Autodesk Inventor part; units mm, degrees
ref_plane "YZ Plane" through (0, 0, 0) normal (1, 0, 0) x (0, 1, 0)
ref_plane "XZ Plane" through (0, 0, 0) normal (0, 1, 0) x (-1, 0, 0)
ref_plane "XY Plane" through (0, 0, 0) normal (0, 0, 1) x (1, 0, 0)
ref_plane "РабПлоскость1" through (51.8181, -3.2568, 14.8616) normal (0, 0, 1) x (1, 0, 0)
sketch "Эскиз1" plane through (51.8181, -3.2568, 14.8616) normal (0, 0, 1) x (1, 0, 0)
  line L0 (-26.6721, 3.7827) -> (-26.6721, -9.7173)
  line L1 (-30.7721, 8.2755) -> (-13.9721, 8.2755)
  line L2 (-13.9721, 8.2755) -> (-13.9721, -14.4178)
  line L3 (-13.9721, -14.4178) -> (-30.7721, -14.4178)
  line L4 (-30.7721, -14.4178) -> (-30.7721, 8.2755)
  point P0 (-51.8181, 3.2568)
extrude "Выдавливание1" add sketch "Эскиз1" along normal blind 3
sketch "Эскиз2" plane through (51.8181, -3.2568, 14.8616) normal (0, 0, -1) x (-1, 0, 0)
  circle A0 centre (27.4758, 1.0327) radius 1.2
  circle A1 centre (15.4758, 1.0327) radius 1.2
  circle A2 centre (15.4758, -6.9673) radius 1.2
  circle A3 centre (27.4758, -6.9673) radius 1.2
  point P0 (51.8181, 3.2568)
extrude "Выдавливание2" cut sketch "Эскиз2" against normal blind 10
sketch "Эскиз3" plane through (51.8181, -3.2568, 14.8616) normal (0, 0, -1) x (-1, 0, 0)
  line L0 (30.7721, -14.4178) -> (13.9721, -14.4178)
  line L1 (13.9721, -14.4178) -> (28.9801, -14.4178)
  line L2 (28.9801, -14.4178) -> (28.9801, 8.2755)
  line L3 (28.9801, 8.2755) -> (13.9721, 8.2755)
  line L4 (13.9721, 8.2755) -> (13.9721, -14.4178)
  line L5 (13.9721, 8.2755) -> (30.7721, 8.2755)
  line L6 (30.7721, -14.4178) -> (28.9801, -14.4178)
  line L7 (28.9801, -14.4178) -> (28.9801, 8.2755)
  line L8 (28.9801, 8.2755) -> (30.7721, 8.2755)
  line L9 (30.7721, 8.2755) -> (30.7721, -14.4178)
  point P0 (51.8181, 3.2568)
  point P1 (30.7721, 8.2755)
  point P2 (28.9801, 8.2755)
  dimension "d4" = 15.008
extrude "Выдавливание3" cut sketch "Эскиз3" against normal blind 10 contours L0 L2 L5 L9
properties part number "проставк"
Model file for the job. Use its own axes, mm. Give positions to 0.01 mm unless a question says otherwise; leave off trailing zeros. Order: outer loops, then holes, each group sorted by start corner. A loop starts at its lowest first (then second) coordinate and runs counter-clockwise, first axis right, second up. Notation, with made-up numbers: M -5.75,13 L 34.25,13 A21 ccw 34.25,32 Z; hole C 15.25,13.25 d2. An arc over 180 degrees is marked long. Write item = value, one per line.
Q1. Cut at B-B, the plane z = 16.55. List the corners of the cut face in (x, y), then the cut area to 3 significant figures.
Derived:
outline = M 22.84,-17.67 L 37.85,-17.67 L 37.85,5.02 L 22.84,5.02 Z; hole C 24.34,-10.22 d2.4; hole C 24.34,-2.22 d2.4; hole C 36.34,-10.22 d2.4; hole C 36.34,-2.22 d2.4
area = 322 mm2
Q2. Cut at C-C, the plane y = -10.75. List the corners of the cut face in (x, z).
Derived:
outline = M 22.84,14.86 L 23.26,14.86 L 23.26,17.86 L 22.84,17.86 Z; M 25.42,14.86 L 35.26,14.86 L 35.26,17.86 L 25.42,17.86 Z; M 37.42,14.86 L 37.85,14.86 L 37.85,17.86 L 37.42,17.86 Z
Q3. Cut at A-A, the plane x = 35.5. List the corners of the cut face in (y, z), then the cut area to 3 significant figures.
Derived:
outline = M -17.67,14.86 L -11.08,14.86 L -11.08,17.86 L -17.67,17.86 Z; M -9.37,14.86 L -3.08,14.86 L -3.08,17.86 L -9.37,17.86 Z; M -1.37,14.86 L 5.02,14.86 L 5.02,17.86 L -1.37,17.86 Z
area = 57.8 mm2
Q4. Drill centre lines: line 1 (Y direction, x = 24.25, z = 15.85); line 2 (Y direction, x = 25, z = 16.9); line 3 (X direction, y = -10.5, z = 15.2). Where is each one in solid material? Low to high. Write a range as [from, to].
Derived:
line_1 = [-17.67, -11.42], [-9.03, -3.42], [-1.03, 5.02]
line_2 = [-17.67, -11.23], [-9.22, -3.23], [-1.22, 5.02]
line_3 = [22.84, 23.17], [25.51, 35.17], [37.51, 37.85]
Q5. Two-plate mould, pull along Y, no slides. Class faces 1 (the flat face through (30, -6, 14.862)), 2 (the flat face through (30, -17.675, 16)), 3 (the cylindrical face through (37.54, -2.17, 16.34)), 4 (the flat face through (30, 5.019, 16)): pulls with the +Y half, pulls with the -Y half, needs draft (parallel to the pull), parting line crosses it, or undercut.
Derived:
face_1 = needs draft
face_2 = pulls with the -Y half
face_3 = undercut
face_4 = pulls with the +Y half
